CAD build for the part. Positions are in the model's coordinates, mm. Coordinates: 2 decimals unless noted, no trailing zeros. Loops run counter-clockwise (first coordinate to the right, second up) from the corner with the lowest first, then second, coordinate; pieces in that order, holes last.
1) Saw through at D-D, the plane x = -32. Write the cut outline in (y, z).
2) Saw through at B-B, the plane z = -61. Write the cut outline in (x, y).
3) Saw through at C-C, the plane z = 8. Write the cut outline in (x, y).
4) Saw through at A-A, the plane y = 7.25. Give the number of separate pieces and of enclosed holes in the cut face, and give its area (3 significant figures).
5) Wall check: line 1 along X through (y, z) = (3.5, -61); line 2 along X through (y, z) = (4, -45.5); line 3 along X through (y, z) = (7.25, 8). Give the ranges that are in metal, low to high.
6) Pin check, flat tips, straight feed: pin 1 Ø4 at (x, z) = (-15, 8) entering from +Y; pin 2 Ø5 at (x, y) = (-45.5, 4) entering from +Z. Stop position of each tip, or through.
```python
from build123d import *

# Parameters (mm, degrees)
SKETCH1_W           = 60
SKETCH1_H           = 140
BOSS_EXTRUDE1_DEPTH = 10
SKETCH3_R           = 1.55
CUT_EXTRUDE1_DEPTH  = 77.811457479
SKETCH4_R           = 1.55
CUT_EXTRUDE2_DEPTH  = 77.811457479
SKETCH7_W           = 25
SKETCH7_H           = 90
BOSS_EXTRUDE2_DEPTH = 10
SKETCH8_R           = 1.55
SKETCH8_R_2         = 12.5
CUT_EXTRUDE4_DEPTH  = 90.582364336
SKETCH9_W           = 30
SKETCH9_H           = 90
BOSS_EXTRUDE3_DEPTH = 10
SKETCH10_R          = 1.55
SKETCH10_R_2        = 12.5
CUT_EXTRUDE5_DEPTH  = 93.736184955
SKETCH11_R          = 2.5
CUT_EXTRUDE6_DEPTH  = 93.736184955
SKETCH12_R          = 1.1
CUT_EXTRUDE7_DEPTH  = 93.736184955
CUT_EXTRUDE8_REACH  = 94.736
SKETCH13_R          = 1.1


with BuildPart() as part:
    # Sketch1 → Boss-Extrude1 (new body)
    with BuildSketch(Plane(origin=(0, 0, 0), x_dir=(1, 0, 0), z_dir=(0, 1, 0))):
        Rectangle(SKETCH1_W, SKETCH1_H)
    extrude(amount=BOSS_EXTRUDE1_DEPTH)

    # Sketch3 → Cut-Extrude1 (cut, through all)
    with BuildSketch(Plane(origin=(0, 10, 0), x_dir=(1, 0, 0), z_dir=(0, 1, 0))):
        with Locations(Location((0, -60, 0), (0, 0, 270))):
            Circle(SKETCH3_R)
        with Locations(Location((0, -20, 0), (0, 0, 270))):
            Circle(SKETCH3_R)
        with Locations(Location((0, 20, 0), (0, 0, 270))):
            Circle(SKETCH3_R)
    extrude(amount=-CUT_EXTRUDE1_DEPTH, mode=Mode.SUBTRACT)

    # Sketch4 → Cut-Extrude2 (cut, through all)
    with BuildSketch(Plane(origin=(0, 10, 0), x_dir=(1, 0, 0), z_dir=(0, 1, 0))):
        with Locations(Location((12.5, -27.5, 0), (0, 0, 270))):
            Circle(SKETCH4_R)
        with Locations(Location((12.5, -52.5, 0), (0, 0, 270))):
            Circle(SKETCH4_R)
        with Locations(Location((-12.5, -27.5, 0), (0, 0, 270))):
            Circle(SKETCH4_R)
        with Locations(Location((-12.5, -52.5, 0), (0, 0, 270))):
            Circle(SKETCH4_R)
    extrude(amount=-CUT_EXTRUDE2_DEPTH, mode=Mode.SUBTRACT)

    # Sketch7 → Boss-Extrude2 (add)
    with BuildSketch(Plane(origin=(0, 10, 0), x_dir=(1, 0, 0), z_dir=(0, 1, 0))):
        with Locations((42.5, 25)):
            Rectangle(SKETCH7_W, SKETCH7_H)
    extrude(amount=-BOSS_EXTRUDE2_DEPTH)

    # Sketch8 → Cut-Extrude4 (cut, through all)
    with BuildSketch(Plane(origin=(0, 10, 0), x_dir=(1, 0, 0), z_dir=(0, 1, 0))):
        with Locations(Location((14, 30, 0), (0, 0, 270))):
            Circle(SKETCH8_R)
        with Locations(Location((45, 30, 0), (0, 0, 270))):
            Circle(SKETCH8_R)
        with Locations(Location((45, 61, 0), (0, 0, 270))):
            Circle(SKETCH8_R)
        with Locations(Location((14, 61, 0), (0, 0, 270))):
            Circle(SKETCH8_R)
        with Locations(Location((29.5, 45.5, 0), (0, 0, 270))):
            Circle(SKETCH8_R_2)
    extrude(amount=-CUT_EXTRUDE4_DEPTH, mode=Mode.SUBTRACT)

    # Sketch9 → Boss-Extrude3 (add)
    with BuildSketch(Plane(origin=(0, 10, 0), x_dir=(1, 0, 0), z_dir=(0, 1, 0))):
        with Locations((-45, 25)):
            Rectangle(SKETCH9_W, SKETCH9_H)
    extrude(amount=-BOSS_EXTRUDE3_DEPTH)

    # Sketch10 → Cut-Extrude5 (cut, through all)
    with BuildSketch(Plane(origin=(0, 10, 0), x_dir=(1, 0, 0), z_dir=(0, 1, 0))):
        with Locations(Location((-47.5, 61, 0), (0, 0, 270))):
            Circle(SKETCH10_R)
        with Locations(Location((-16.5, 61, 0), (0, 0, 270))):
            Circle(SKETCH10_R)
        with Locations(Location((-16.5, 30, 0), (0, 0, 270))):
            Circle(SKETCH10_R)
        with Locations(Location((-47.5, 30, 0), (0, 0, 270))):
            Circle(SKETCH10_R)
        with Locations(Location((-32, 45.5, 0), (0, 0, 270))):
            Circle(SKETCH10_R_2)
    extrude(amount=-CUT_EXTRUDE5_DEPTH, mode=Mode.SUBTRACT)

    # Sketch11 → Cut-Extrude6 (cut, through all)
    with BuildSketch(Plane(origin=(0, 10, 0), x_dir=(1, 0, 0), z_dir=(0, 1, 0))):
        with Locations(Location((-44, -8, 0), (0, 0, 270))):
            Circle(SKETCH11_R)
        with Locations(Location((-15, -8, 0), (0, 0, 270))):
            Circle(SKETCH11_R)
    extrude(amount=-CUT_EXTRUDE6_DEPTH, mode=Mode.SUBTRACT)

    # Sketch12 → Cut-Extrude7 (cut, through all)
    with BuildSketch(Plane(origin=(0, 10, 0), x_dir=(1, 0, 0), z_dir=(0, 1, 0))):
        with Locations(Location((-24.5, -60, 0), (0, 0, 270))):
            Circle(SKETCH12_R)
        with Locations(Location((-15, -60, 0), (0, 0, 270))):
            Circle(SKETCH12_R)
    extrude(amount=-CUT_EXTRUDE7_DEPTH, mode=Mode.SUBTRACT)

    # Sketch13 → Cut-Extrude8 (cut, up to next)
    with BuildSketch(Plane.XZ, mode=Mode.PRIVATE) as cut_extrude8_sk1:
        with Locations(Location((33, -9.5, 0), (0, 0, 270))):
            Circle(SKETCH13_R)
    cut_extrude8_tool1 = extrude(cut_extrude8_sk1.sketch, amount=-CUT_EXTRUDE8_REACH, mode=Mode.PRIVATE) & part.part
    # Sketch13 → Cut-Extrude8 (cut, up to next)
    with BuildSketch(Plane.XZ, mode=Mode.PRIVATE) as cut_extrude8_sk2:
        with Locations(Location((33, 0, 0), (0, 0, 270))):
            Circle(SKETCH13_R)
    cut_extrude8_tool2 = extrude(cut_extrude8_sk2.sketch, amount=-CUT_EXTRUDE8_REACH, mode=Mode.PRIVATE) & part.part
    add(cut_extrude8_tool1.solids().sort_by_distance((33, 0, -9.5))[0], mode=Mode.SUBTRACT)
    add(cut_extrude8_tool2.solids().sort_by_distance((33, 0, 0))[0], mode=Mode.SUBTRACT)


solid = part.part
```
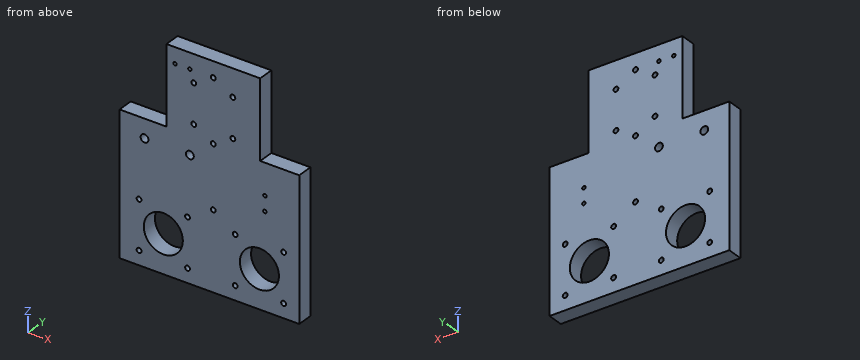
Data:
1. outline: (0, -70) - (10, -70) - (10, -58) - (0, -58) - close; (0, -33) - (10, -33) - (10, 20) - (0, 20) - close
2. outline: (-60, 0) - (-49.05, 0) - (-49.05, 10) - (-60, 10) - close; (-45.95, 0) - (-18.05, 0) - (-18.05, 10) - (-45.95, 10) - close; (-14.95, 0) - (12.45, 0) - (12.45, 10) - (-14.95, 10) - close; (15.55, 0) - (43.45, 0) - (43.45, 10) - (15.55, 10) - close; (46.55, 0) - (55, 0) - (55, 10) - (46.55, 10) - close
3. outline: (-60, 0) - (-46.5, 0) - (-46.5, 10) - (-60, 10) - close; (-41.5, 0) - (-17.5, 0) - (-17.5, 10) - (-41.5, 10) - close; (-12.5, 0) - (55, 0) - (55, 10) - (-12.5, 10) - close
4. separate pieces: 1
4. enclosed holes: 23
4. area: 12,200 mm2
5. line 1: x = -60 to -49.05, -45.95 to -18.05, -14.95 to 12.45, 15.55 to 43.45, 46.55 to 55
5. line 2: x = -60 to -44.5, -19.5 to 17, 42 to 55
5. line 3: x = -60 to -46.5, -41.5 to -17.5, -12.5 to 55
6. pin 1: passes through
6. pin 2: stops at z = 20
